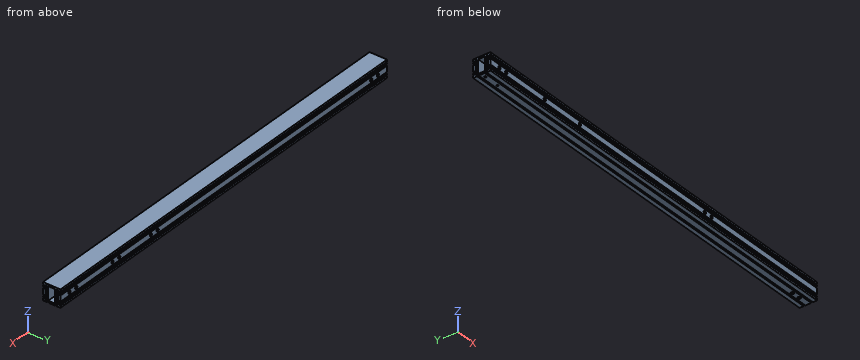
from build123d import *

# Parameters (mm, degrees)
SKETCH_1_W             = 23.5
SKETCH_1_H             = 12
EXTRUDE_1_DEPTH        = 361
HOLE_WIZARD_M6_1_D     = 5
HOLE_WIZARD_M6_1_DEPTH = 19
HOLE_WIZARD_M6_1_TIP   = 1.502151548
HOLE_WIZARD_M6_2_D     = 5
HOLE_WIZARD_M6_2_DEPTH = 19
HOLE_WIZARD_M6_2_TIP   = 1.502151548
HOLE_WIZARD_M4_1_D     = 3.3
HOLE_WIZARD_M4_1_DEPTH = 11.5
HOLE_WIZARD_M4_1_TIP   = 0.991420021
HOLE_WIZARD_M6_4_D     = 5
HOLE_WIZARD_M6_4_DEPTH = 19
HOLE_WIZARD_M6_4_TIP   = 1.502151548


with BuildPart() as part:
    # 草图1 → 凸台-拉伸1 (new, symmetric)
    with BuildSketch(Plane(origin=(0, 0, 0), x_dir=(0, 0, -1), z_dir=(1, 0, 0))):
        Polygon((-15, 15), (-11.5, 15), (-11.5, 13.5), (-11, 13.5), (-11, 12), (-9.5, 12), (-9.5, 15), (-8, 15), (-8, 12.5), (-5, 12.5), (-5, 15), (5, 15), (5, 12.5), (8, 12.5), (8, 15), (9.5, 15), (9.5, 12), (11, 12), (11, 13.5), (11.5, 13.5), (11.5, 15), (15, 15), (15, 8), (12.5, 8), (12.5, 5), (15, 5), (15, -5), (12.5, -5), (12.5, -8), (15, -8), (15, -15), (11.5, -15), (11.5, -13.5), (11, -13.5), (11, -12), (9.5, -12), (9.5, -15), (8, -15), (8, -12.5), (5, -12.5), (5, -15), (-5, -15), (-5, -12.5), (-8, -12.5), (-8, -15), (-9.5, -15), (-9.5, -12), (-11, -12), (-11, -13.5), (-11.5, -13.5), (-11.5, -15), (-15, -15), align=None)
        with BuildLine():
            Line((12, -10.5), (12, -8.5))
            ThreePointArc((12, -8.5), (11.853553391, -8.146446609), (11.5, -8))
            Line((11.5, -8), (-11.5, -8))
            ThreePointArc((-11.5, -8), (-11.853553391, -8.146446609), (-12, -8.5))
            Line((-12, -8.5), (-12, -10.5))
            ThreePointArc((-12, -10.5), (-11.853553391, -10.853553391), (-11.5, -11))
            Line((-11.5, -11), (11.5, -11))
            ThreePointArc((11.5, -11), (11.853553391, -10.853553391), (12, -10.5))
        make_face(mode=Mode.SUBTRACT)
        with BuildLine():
            Line((-11.5, 11), (11.5, 11))
            ThreePointArc((11.5, 11), (11.853553391, 10.853553391), (12, 10.5))
            Line((12, 10.5), (12, 8.5))
            ThreePointArc((12, 8.5), (11.853553391, 8.146446609), (11.5, 8))
            Line((11.5, 8), (-11.5, 8))
            ThreePointArc((-11.5, 8), (-11.853553391, 8.146446609), (-12, 8.5))
            Line((-12, 8.5), (-12, 10.5))
            ThreePointArc((-12, 10.5), (-11.853553391, 10.853553391), (-11.5, 11))
        make_face(mode=Mode.SUBTRACT)
        Rectangle(SKETCH_1_W, SKETCH_1_H, mode=Mode.SUBTRACT)
    extrude(amount=EXTRUDE_1_DEPTH, both=True)

    # M6 螺纹孔1
    with Locations(Plane(origin=(0, 15, 0), x_dir=(1, 0, 0), z_dir=(0, 1, 0))):
        with Locations((341, 0), (326, 0), (246, 0), (231, 0), (161, 0), (146, 0), (-326, 0), (-341, 0)):
            Hole(HOLE_WIZARD_M6_1_D / 2, depth=HOLE_WIZARD_M6_1_DEPTH)
            with Locations((0, 0, -(HOLE_WIZARD_M6_1_DEPTH + HOLE_WIZARD_M6_1_TIP / 2))):  # 118° drill point
                Cone(0, HOLE_WIZARD_M6_1_D / 2, HOLE_WIZARD_M6_1_TIP, mode=Mode.SUBTRACT)

    # M6 螺纹孔2
    with Locations(Plane(origin=(0, -15, 0), x_dir=(-1, 0, 0), z_dir=(0, -1, 0))):
        with Locations((-128, 0), (-113, 0), (326, 0), (341, 0), (241, 0), (163, 0)):
            Hole(HOLE_WIZARD_M6_2_D / 2, depth=HOLE_WIZARD_M6_2_DEPTH)
            with Locations((0, 0, -(HOLE_WIZARD_M6_2_DEPTH + HOLE_WIZARD_M6_2_TIP / 2))):  # 118° drill point
                Cone(0, HOLE_WIZARD_M6_2_D / 2, HOLE_WIZARD_M6_2_TIP, mode=Mode.SUBTRACT)

    # M4 螺纹孔1
    with Locations(Plane(origin=(0, 0, -15), x_dir=(-1, 0, 0), z_dir=(0, 0, -1))):
        with Locations((353, 0), (326, 0)):
            Hole(HOLE_WIZARD_M4_1_D / 2, depth=HOLE_WIZARD_M4_1_DEPTH)
            with Locations((0, 0, -(HOLE_WIZARD_M4_1_DEPTH + HOLE_WIZARD_M4_1_TIP / 2))):  # 118° drill point
                Cone(0, HOLE_WIZARD_M4_1_D / 2, HOLE_WIZARD_M4_1_TIP, mode=Mode.SUBTRACT)

    # M6 螺纹孔4
    with Locations(Plane(origin=(0, 0, -15), x_dir=(-1, 0, 0), z_dir=(0, 0, -1))):
        with Locations((-326, 0), (-341, 0)):
            Hole(HOLE_WIZARD_M6_4_D / 2, depth=HOLE_WIZARD_M6_4_DEPTH)
            with Locations((0, 0, -(HOLE_WIZARD_M6_4_DEPTH + HOLE_WIZARD_M6_4_TIP / 2))):  # 118° drill point
                Cone(0, HOLE_WIZARD_M6_4_D / 2, HOLE_WIZARD_M6_4_TIP, mode=Mode.SUBTRACT)


solid = part.part
Can you work these out from the model? Positions are in its coordinate system, mm. Round coordinates to 2 decimals unless told otherwise and drop trailing zeros. One line per question, with ' | ' between items. Start each with the question number.
1) Suppose I cut it at A-A on x = 195. Count the separate pieces of the cut face and the enclosed holes in it, then the cut area to 3 significant figures.
2) I'm going to push flat-ended pins straight in: P1, Ø1.5, axis at y = 9.5, z = -11.5, coming from the -X side; P2, Ø4.5, axis at x = -341, z = 0, coming from the -Y side; P3, Ø1.5, axis at x = -26.5, y = -7, coming from the -Z side. Where does each tip first touch, or does it pass through?
3) I need wall thicknesses on line 1 (Y direction, x = 13, z = -6); line 2 (Z direction, x = 326, y = 12.3); line 3 (Y direction, x = 13, z = -13). Which ranges of each line are inside material? Lowest first, please. Write a range as [from, to].
Return value:
1) separate pieces: 1 | enclosed holes: 3 | area: 408 mm2
2) P1: stops at x = -361 | P2: passes through | P3: stops at z = -12.5
3) line 1: y = [-12.5, -11], [-8, -6], [6, 8], [11, 12.5] | line 2: z = [-15, -11], [-9.5, -2.5], [2.5, 9.5], [11, 15] | line 3: y = [-15, -8], [-5, 5], [8, 15]
